```python
from build123d import *

# Parameters (mm, degrees)
SKETCH_1_R      = 1
SKETCH_1_R_2    = 2
SKETCH_1_W      = 12
SKETCH_1_H      = 23
EXTRUDE_1_DEPTH = 3


with BuildPart() as part:
    # 草图1 → 凸台-拉伸1 (new body)
    with BuildSketch(Plane.XY):
        with BuildLine():
            Line((32, -8), (32, -11.464101615))
            ThreePointArc((32, -11.464101615), (32.068166714, -11.981729308), (32.268018761, -12.464061443))
            Line((32.268018761, -12.464061443), (35.500063979, -18.060190477))
            ThreePointArc((35.500063979, -18.060190477), (36.232094687, -18.7920566), (37.231964862, -19.059930845))
            Line((37.231964862, -19.059930845), (44.515960818, -19.059930845))
            ThreePointArc((44.515960818, -19.059930845), (45.93017438, -18.474144407), (46.515960818, -17.059930845))
            Line((46.515960818, -17.059930845), (46.515960818, -17))
            ThreePointArc((46.515960818, -17), (47.101747256, -15.585786438), (48.515960818, -15))
            Line((48.515960818, -15), (51, -15))
            ThreePointArc((51, -15), (56.656854249, -12.656854249), (59, -7))
            Line((59, -7), (59, -5))
            ThreePointArc((59, -5), (57.535533906, -1.464466094), (54, 0))
            ThreePointArc((54, 0), (50.464466094, 1.464466094), (49, 5))
            Line((49, 5), (49, 10))
            ThreePointArc((49, 10), (47.535533906, 13.535533906), (44, 15))
            Line((44, 15), (-18, 15))
            ThreePointArc((-18, 15), (-23.656854249, 12.656854249), (-26, 7))
            Line((-26, 7), (-26, -2))
            ThreePointArc((-26, -2), (-25.121320344, -4.121320344), (-23, -5))
            Line((-23, -5), (28.999778597, -4.924134531))
            ThreePointArc((28.999778597, -4.924134531), (31.148522662, -5.829385596), (32, -8))
        make_face()
        with Locations((-20.828427125, 9.828427125)):
            Circle(SKETCH_1_R, mode=Mode.SUBTRACT)
        Circle(SKETCH_1_R_2, mode=Mode.SUBTRACT)
        with Locations((22.627416998, 8)):
            Circle(SKETCH_1_R_2, mode=Mode.SUBTRACT)
        with Locations((37.265960818, 11.5)):
            Circle(SKETCH_1_R, mode=Mode.SUBTRACT)
        with Locations((43.765960818, 11.5)):
            Circle(SKETCH_1_R, mode=Mode.SUBTRACT)
        with Locations((54, -5)):
            Circle(SKETCH_1_R, mode=Mode.SUBTRACT)
        with Locations(Location((43.765960818, -16.5, 0), (0, 0, 180))):
            Circle(SKETCH_1_R, mode=Mode.SUBTRACT)
        with Locations(Location((37.265960818, -16.5, 0), (0, 0, 180))):
            Circle(SKETCH_1_R, mode=Mode.SUBTRACT)
        with Locations((40.515960818, -2.5)):
            Rectangle(SKETCH_1_W, SKETCH_1_H, mode=Mode.SUBTRACT)
        with BuildLine():
            Line((-21.865827163, 2.988199444), (8.016167282, 5.646471071))
            ThreePointArc((8.016167282, 5.646471071), (8.666972603, 5.101996614), (8.122498147, 4.451191293))
            Line((8.122498147, 4.451191293), (-18.522663358, 2.08086501))
            ThreePointArc((-18.522663358, 2.08086501), (-18.915607181, 1.825347502), (-18.924307569, 1.356712945))
            ThreePointArc((-18.924307569, 1.356712945), (-23.055094396, -2.623490099), (-21.865827163, 2.988199444))
        make_face(mode=Mode.SUBTRACT)
    extrude(amount=EXTRUDE_1_DEPTH)


solid = part.part
```
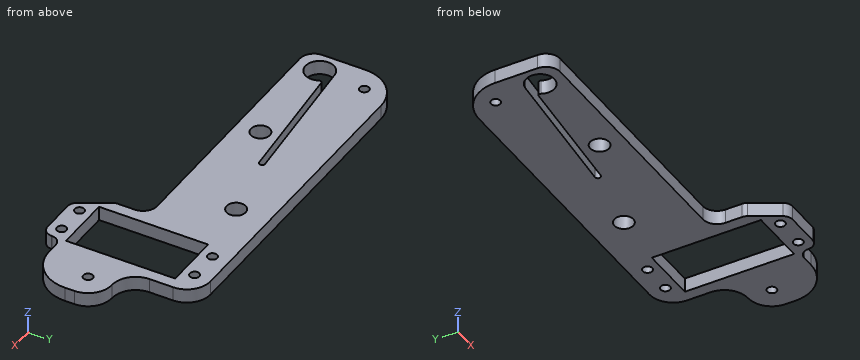
Geometry check sheet. Reference: the model listing, model coordinates, mm. Coordinates: 2 decimals unless noted, no trailing zeros. Order: outer loops, then holes, each group sorted by start corner. A loop starts at its lowest first (then second) coordinate and runs counter-clockwise, first axis right, second up. Notation, with made-up numbers: M -3.5,55 L 26.5,55 A25 cw 26.5,68 Z; hole C -5.75,31 d8. An arc over 180 degrees is marked long. One line per question, with ' | ' between items. Start each with the question number.
Item 1: Cross-section at D-D on x = 23. Enter the section's corners in (y, z), then the cut area to 3 significant figures.
Item 2: Cross-section at B-B on x = 0. Enter the section's corners in (y, z), then the cut area to 3 significant figures.
Item 3: Cross-section at C-C on y = -9. Enter the section's corners in (x, z), then the cut area to 3 significant figures.
Item 4: Cross-section at A-A on y = 8. Enter the section's corners in (x, z).
Item 5: Material ranges on L1, parallel to Y at x = -21.6, z = 2.4; L2, parallel to Y at x = 42, z = 0.25; L3, parallel to X at y = -5.5, z = 0.55, recorded low to high. Write a range as [from, to].
Item 6: Gauge pin test, flat ends, axial feed: pin 1 (0.7 mm diameter, centred on x = 50, z = 2, fed in from -Y); pin 2 (1.6 mm diameter, centred on x = 43.77, y = 11.5, fed in from -Z); pin 3 (0.9 mm diameter, centred on y = 8, z = 2, fed in from +X); pin 4 (1.5 mm diameter, centred on x = 45.5, z = 0.5, fed in from +Y). Record the tip position at first contact, or that the pin passes through.
Findings:
1) outline: M -4.93,0 L 6.04,0 L 6.04,3 L -4.93,3 Z; M 9.96,0 L 15,0 L 15,3 L 9.96,3 Z | area: 48.0 mm²
2) outline: M -4.97,0 L -2,0 L -2,3 L -4.97,3 Z; M 2,0 L 3.73,0 L 3.73,3 L 2,3 Z; M 4.93,0 L 15,0 L 15,3 L 4.93,3 Z | area: 44.3 mm²
3) outline: M 32,0 L 34.52,0 L 34.52,3 L 32,3 Z; M 46.52,0 L 58.75,0 L 58.75,3 L 46.52,3 Z | area: 44.2 mm²
4) outline: M -25.94,0 L 20.63,0 L 20.63,3 L -25.94,3 Z; M 24.63,0 L 34.52,0 L 34.52,3 L 24.63,3 Z; M 46.52,0 L 49,0 L 49,3 L 46.52,3 Z
5) L1: y = [-5, -3], [3.01, 9.19], [10.46, 14.14] | L2: y = [-19.06, -14], [9, 15] | L3: x = [30.77, 34.52], [46.52, 53.13], [54.87, 59]
6) pin 1: stops at y = -15 | pin 2: passes through | pin 3: stops at x = 49 | pin 4: stops at y = 14.94
